CAD build for the part. Positions are in the model's coordinates, mm. A direction names the side the tool comes from. Give positions to 0.01 mm unless a question says otherwise; leave off trailing zeros. Write each loop counter-clockwise with the first axis right and the second up, starting at its lowest first coordinate (ties: lowest second). Pieces come first, ordered by that corner, then holes. Notation, with made-up numbers: (-4.5, 47) -> (3.5, 47) arc R13 cw to (3.5, 51) -> close; hole circle Ø6 at (22.25, 60.5). An arc over 180 degrees is marked (long way). Answer in a Markdown table with one row per item. Add a question column.
```python
from build123d import *

# Parameters (mm, degrees)
CYLINDER1267_R              = 1.5
CYLINDER1267_DEPTH          = 32
CYLINDER1266_R              = 1.5
CYLINDER1266_DEPTH          = 32
CYLINDER1265_R              = 1.5
CYLINDER1265_DEPTH          = 100
CYLINDER1264_R              = 1.5
CYLINDER1264_DEPTH          = 100
CYLINDER1259_R              = 3
CYLINDER1259_DEPTH          = 3
CYLINDER1258_R              = 3
CYLINDER1258_DEPTH          = 3
CYLINDER581_R               = 3
CYLINDER581_DEPTH           = 4
CYLINDER582_R               = 3
CYLINDER582_DEPTH           = 4
CYLINDER580_R               = 3
CYLINDER580_DEPTH           = 4
CYLINDER575_R               = 3
CYLINDER575_DEPTH           = 4
COMPOUND338_PLACEMENT_ANGLE = 90
CYLINDER576_R               = 1.5
CYLINDER576_DEPTH           = 20
CYLINDER578_R               = 1.5
CYLINDER578_DEPTH           = 20
CYLINDER579_R               = 1.5
CYLINDER579_DEPTH           = 20
CYLINDER577_R               = 1.5
CYLINDER577_DEPTH           = 20
COMPOUND337_PLACEMENT_ANGLE = 90
PAD001_DEPTH                = 10


with BuildPart() as obj1:
    # Cylinder1267 → Cylinder1267 (new body)
    with BuildSketch(Plane(origin=(78, 41, -42), x_dir=(1, 0, 0), z_dir=(0, 0, 1))):
        Circle(CYLINDER1267_R)
    extrude(amount=CYLINDER1267_DEPTH)


with BuildPart() as compound649:
    # Cylinder1266 → Cylinder1266 (new body)
    with BuildSketch(Plane(origin=(26, 41, -42), x_dir=(1, 0, 0), z_dir=(0, 0, 1))):
        Circle(CYLINDER1266_R)
    extrude(amount=CYLINDER1266_DEPTH)

    # Compound649: union obj1
    add(obj1.part)


with BuildPart() as compound649_1:
    # Compound649 placement: moved
    add(compound649.part.moved(Location((-52, 0, 36))))


with BuildPart() as obj2:
    # Cylinder1265 → Cylinder1265 (new body)
    with BuildSketch(Plane(origin=(14, 0, -60), x_dir=(1, 0, 0), z_dir=(0, 0, 1))):
        Circle(CYLINDER1265_R)
    extrude(amount=CYLINDER1265_DEPTH)


with BuildPart() as compound647:
    # Cylinder1264 → Cylinder1264 (new body)
    with BuildSketch(Plane(origin=(90, 0, -60), x_dir=(1, 0, 0), z_dir=(0, 0, 1))):
        Circle(CYLINDER1264_R)
    extrude(amount=CYLINDER1264_DEPTH)

    # Compound648: union obj2
    add(obj2.part)


with BuildPart() as compound647_1:
    # Compound648 placement: moved
    add(compound647.part.moved(Location((-52, 0, 0))))

    # Compound647: union Compound649
    add(compound649_1.part)


with BuildPart() as obj3:
    # Cylinder1259 → Cylinder1259 (new body)
    with BuildSketch(Plane(origin=(78, 41, -42), x_dir=(1, 0, 0), z_dir=(0, 0, 1))):
        Circle(CYLINDER1259_R)
    extrude(amount=CYLINDER1259_DEPTH)


with BuildPart() as compound642:
    # Cylinder1258 → Cylinder1258 (new body)
    with BuildSketch(Plane(origin=(26, 41, -42), x_dir=(1, 0, 0), z_dir=(0, 0, 1))):
        Circle(CYLINDER1258_R)
    extrude(amount=CYLINDER1258_DEPTH)

    # Compound642: union obj3
    add(obj3.part)


with BuildPart() as compound642_1:
    # Compound642 placement: moved
    add(compound642.part.moved(Location((-52, 0, 42))))


with BuildPart() as obj4:
    # Cylinder581 → Cylinder581 (new body)
    with BuildSketch(Plane(origin=(-7, -34, 37), x_dir=(1, 0, 0), z_dir=(0, -1, 0))):
        Circle(CYLINDER581_R)
    extrude(amount=CYLINDER581_DEPTH)


with BuildPart() as obj5:
    # Cylinder582 → Cylinder582 (new body)
    with BuildSketch(Plane(origin=(7, -34, 73), x_dir=(1, 0, 0), z_dir=(0, -1, 0))):
        Circle(CYLINDER582_R)
    extrude(amount=CYLINDER582_DEPTH)


with BuildPart() as obj6:
    # Cylinder580 → Cylinder580 (new body)
    with BuildSketch(Plane(origin=(-7, -34, 73), x_dir=(1, 0, 0), z_dir=(0, -1, 0))):
        Circle(CYLINDER580_R)
    extrude(amount=CYLINDER580_DEPTH)


with BuildPart() as compound338:
    # Cylinder575 → Cylinder575 (new body)
    with BuildSketch(Plane(origin=(7, -34, 37), x_dir=(1, 0, 0), z_dir=(0, -1, 0))):
        Circle(CYLINDER575_R)
    extrude(amount=CYLINDER575_DEPTH)

    # Compound338: union obj4, obj5, obj6
    add(obj4.part)
    add(obj5.part)
    add(obj6.part)


with BuildPart() as compound338_1:
    # Compound338 placement: moved
    add(compound338.part.moved(Location((0, 154, 45))).rotate(Axis((0, 154, 45), (1, 0, 0)), COMPOUND338_PLACEMENT_ANGLE))


with BuildPart() as obj7:
    # Cylinder576 → Cylinder576 (new body)
    with BuildSketch(Plane(origin=(-7, -34, 37), x_dir=(1, 0, 0), z_dir=(0, -1, 0))):
        Circle(CYLINDER576_R)
    extrude(amount=CYLINDER576_DEPTH)


with BuildPart() as obj8:
    # Cylinder578 → Cylinder578 (new body)
    with BuildSketch(Plane(origin=(7, -34, 73), x_dir=(1, 0, 0), z_dir=(0, -1, 0))):
        Circle(CYLINDER578_R)
    extrude(amount=CYLINDER578_DEPTH)


with BuildPart() as obj9:
    # Cylinder579 → Cylinder579 (new body)
    with BuildSketch(Plane(origin=(-7, -34, 73), x_dir=(1, 0, 0), z_dir=(0, -1, 0))):
        Circle(CYLINDER579_R)
    extrude(amount=CYLINDER579_DEPTH)


with BuildPart() as compound337:
    # Cylinder577 → Cylinder577 (new body)
    with BuildSketch(Plane(origin=(7, -34, 37), x_dir=(1, 0, 0), z_dir=(0, -1, 0))):
        Circle(CYLINDER577_R)
    extrude(amount=CYLINDER577_DEPTH)

    # Compound337: union obj7, obj8, obj9
    add(obj7.part)
    add(obj8.part)
    add(obj9.part)


with BuildPart() as compound337_1:
    # Compound337 placement: moved
    add(compound337.part.moved(Location((0, 154, 45))).rotate(Axis((0, 154, 45), (1, 0, 0)), COMPOUND337_PLACEMENT_ANGLE))


with BuildPart() as cut204:
    # Sketch001 → Pad001 (new body)
    with BuildSketch(Plane.XY):
        Polygon((-51.883896, 28.015725), (-9.412477, 122.34876), (9.417463, 122.34876), (51.774643, 28.198511), (0, 55.140807), align=None)
    extrude(amount=PAD001_DEPTH)

    # Cut192: cut Compound337
    add(compound337_1.part, mode=Mode.SUBTRACT)

    # Cut193: cut Compound338
    add(compound338_1.part, mode=Mode.SUBTRACT)

    # Cut197: cut Compound642
    add(compound642_1.part, mode=Mode.SUBTRACT)

    # Cut204: cut Compound647
    add(compound647_1.part, mode=Mode.SUBTRACT)


solid = cut204.part
```
Item 1: Mould opens along Y. For faces 5 (the face through (1, 76, 10)), 6 (the face through (8.384, 83.662, 8.521)), 7 (the face through (30.3, 75.93, 4.93)) say: released by +Y, released by -Y, zero draft, split by the parting line, or undercut.
Item 2: Slice it at A-A, the plane z = 8.5. List the corners of the cut face in (x, y), then the cut area to 3 significant figures.
Item 3: Probe L1, parallel to X at y = 81, z = 9.1; L2, parallel to Y at x = -7, z = 3.5; L3, parallel to Y at x = -7, z = 8.5. List the from-to ranges inside material, lowest first. Write a range as from..to.
Item 4: Drop flat-ended pins along their axis: pin 1 Ø2.5 at (x, y) = (-7, 117) entering from +Z; pin 2 Ø2 at (y, z) = (69.5, 5.5) entering from +X; pin 3 Ø4 at (x, z) = (-21.5, 7.5) entering from -Y; pin 4 Ø1.5 at (y, z) = (58, 5) entering from +X. Give the stop position or say it passes through.
Item 5: Which spindle directions (+Z, -Z, +X, -X, +Y, -Y) get a long thin tool onto all of the face, cutting with end or side? Do faces 1 (the face through (1, 76, 0)), 2 (the face through (-5.616, 83.662, 8.521)), 3 (the face through (12.68, 48.543, 4.93)), 4 (the face through (27.44, 43.63, 1.48)). Say none if no direction does.
Item 6: Slice it at B-B, the plane x = -7. List the corners of the cut face in (y, z).
Item 7: Slice it at D-D, the plane y = 117. List the corners of the cut face in (x, z), then the cut area to 3 significant figures.
Item 8: Slice it at C-C, the plane y = 38.5. List the corners of the cut face in (x, z), then the cut area to 3 significant figures.
Answer key:
| question | item | result |
|---|---|---|
| 1 | face 5 | zero draft |
| 1 | face 6 | undercut |
| 1 | face 7 | released by +Y |
| 2 | outline | (-51.88, 28.02) -> (-27.48, 40.77) arc R1.5 cw to (-24.97, 42.09) -> (0, 55.14) -> (25.01, 42.13) arc R1.5 cw to (27.49, 40.84) -> (51.77, 28.2) -> (9.42, 122.35) -> (-9.41, 122.35) -> close; hole circle Ø6 at (-7, 81); hole circle Ø6 at (-7, 117); hole circle Ø6 at (7, 81); hole circle Ø6 at (7, 117) |
| 2 | area | 4,250 mm² |
| 3 | L1 | x = -28.03..-10, -4..4, 10..28.02 |
| 3 | L2 | y = 51.48..79.5, 82.5..115.5, 118.5..122.35 |
| 3 | L3 | y = 51.48..78, 84..114, 120..122.35 |
| 4 | pin 1 | passes through |
| 4 | pin 2 | stops at x = 33.64 |
| 4 | pin 3 | stops at y = 42.85 |
| 4 | pin 4 | stops at x = 38.7 |
| 5 | face 1 | -Z, +X, -X, +Y, -Y |
| 5 | face 2 | +Z |
| 5 | face 3 | +Z, -Z, -Y |
| 5 | face 4 | -Z |
| 6 | outline | (51.48, 0) -> (79.5, 0) -> (79.5, 7) -> (78, 7) -> (78, 10) -> (51.48, 10) -> close; (82.5, 0) -> (115.5, 0) -> (115.5, 7) -> (114, 7) -> (114, 10) -> (84, 10) -> (84, 7) -> (82.5, 7) -> close; (118.5, 0) -> (122.35, 0) -> (122.35, 10) -> (120, 10) -> (120, 7) -> (118.5, 7) -> close |
| 7 | outline | (-11.82, 0) -> (-8.5, 0) -> (-8.5, 7) -> (-10, 7) -> (-10, 10) -> (-11.82, 10) -> close; (-5.5, 0) -> (5.5, 0) -> (5.5, 7) -> (4, 7) -> (4, 10) -> (-4, 10) -> (-4, 7) -> (-5.5, 7) -> close; (8.5, 0) -> (11.82, 0) -> (11.82, 10) -> (10, 10) -> (10, 7) -> (8.5, 7) -> close |
| 7 | area | 158 mm² |
| 8 | outline | (-47.16, 0) -> (-31.83, 0) -> (-31.83, 10) -> (-47.16, 10) -> close; (31.98, 0) -> (47.14, 0) -> (47.14, 10) -> (31.98, 10) -> close |
| 8 | area | 305 mm² |
